Job drawing, mm, ordinate dimensions from the low corner. One solid piece. A direction names the side the tool comes from. Coordinates: 2 decimals unless noted, no trailing zeros. Loops run counter-clockwise (first coordinate to the right, second up) from the corner with the lowest first, then second, coordinate; pieces in that order, holes last. Notation, with made-up numbers: (41, 8) - (49, 8) arc R22 cw to (49, 17) - close; hole circle Ø3 at (35.5, 87.5). An arc over 180 degrees is marked (long way). Use a Markdown table: item, result. Add a question column.
1. Band-saw the part on C-C, the plane x = 8.75. Give the cut face in (y, z), plus the area to 3 significant figures.
2. 3-axis set-ups, long thin cutter, end or side, ignore diameter. For the marked faces 1, 2, 3 and 4: which of +Z, -Z, +X, -X, +Y, -Y reach the whole face in a straight line?
3. Wall check: probe 1 along Y at (x, z) = (6.75, 2.75); probe 2 along Y at (x, z) = (13, 6.5); probe 3 along Z at (x, y) = (8.5, 21) (3 decimals). Give the ranges that are in metal, low to high. Write a range as [from, to].
4. Band-saw the part on A-A, the plane y = 10.25. Give the cut face in (x, z).
5. Drop flat-ended pins along their axis: pin 1 (2 mm diameter, centred on x = 10, y = 25, fed in from -Z) (3 decimals); pin 2 (1.8 mm diameter, centred on x = 8, y = 9.5, fed in from +Z); pin 3 (4 mm diameter, centred on x = 9, y = 8, fed in from -Z). Give the stop position or say it passes through.
6. Band-saw the part on B-B, the plane z = 14. Give the cut face in (x, y), plus the area to 3 significant figures.
7. Band-saw the part on D-D, the plane z = 6.5. Give the cut face in (x, y).
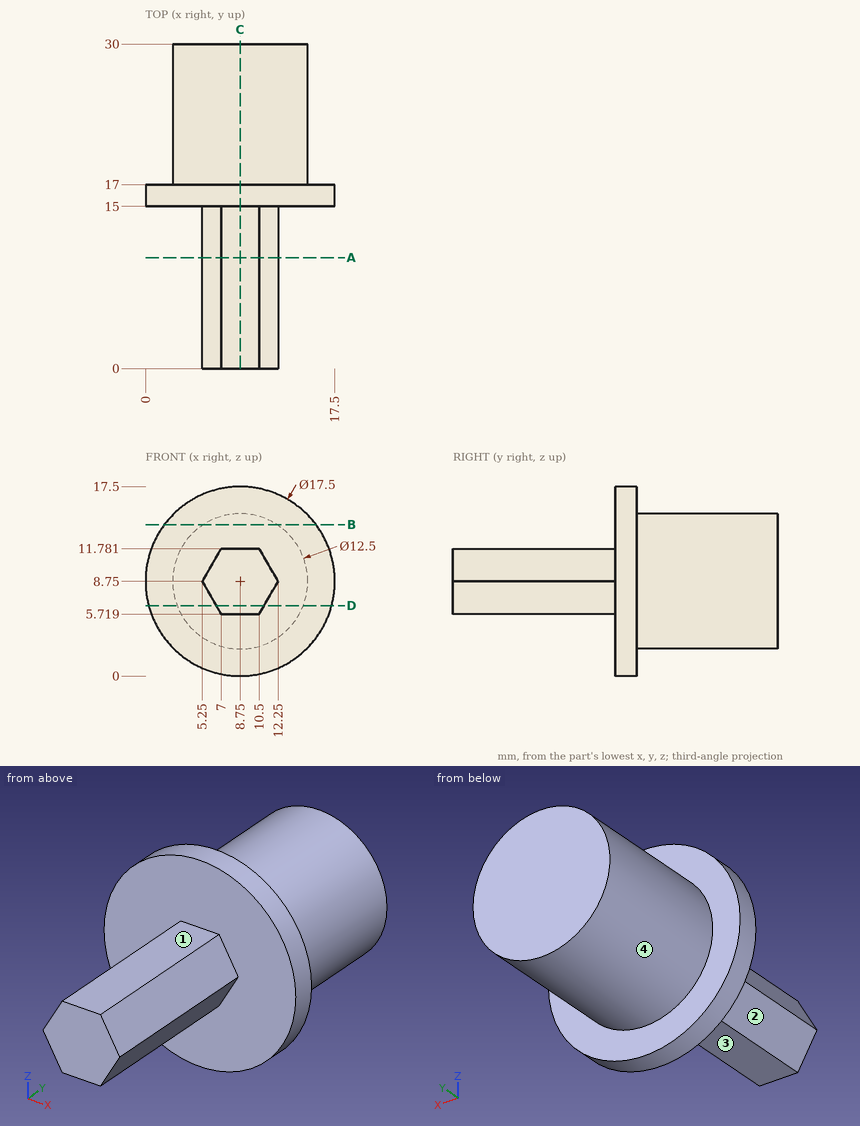
Geometry check:
| question | item | result |
|---|---|---|
| 1 | outline | (0, 5.72) - (15, 5.72) - (15, 0) - (17, 0) - (17, 2.5) - (30, 2.5) - (30, 15) - (17, 15) - (17, 17.5) - (15, 17.5) - (15, 11.78) - (0, 11.78) - close |
| 1 | area | 288 mm^2 |
| 2 | face 1 | +Z, +X, -X, -Y |
| 2 | face 2 | -Z, -X, -Y |
| 2 | face 3 | -Z, +X, -X, -Y |
| 2 | face 4 | +Y |
| 3 | probe 1 | y = [15, 17] |
| 3 | probe 2 | y = [15, 30] |
| 3 | probe 3 | z = [2.505, 14.995] |
| 4 | outline | (5.25, 8.75) - (7, 5.72) - (10.5, 5.72) - (12.25, 8.75) - (10.5, 11.78) - (7, 11.78) - close |
| 5 | pin 1 | stops at z = 2.505 |
| 5 | pin 2 | stops at z = 11.78 |
| 5 | pin 3 | stops at z = 5.72 |
| 6 | outline | (1.75, 15) - (15.75, 15) - (15.75, 17) - (12.14, 17) - (12.14, 30) - (5.36, 30) - (5.36, 17) - (1.75, 17) - close |
| 6 | area | 116 mm^2 |
| 7 | outline | (0.29, 15) - (6.55, 15) - (6.55, 0) - (10.95, 0) - (10.95, 15) - (17.21, 15) - (17.21, 17) - (14.58, 17) - (14.58, 30) - (2.92, 30) - (2.92, 17) - (0.29, 17) - close |
